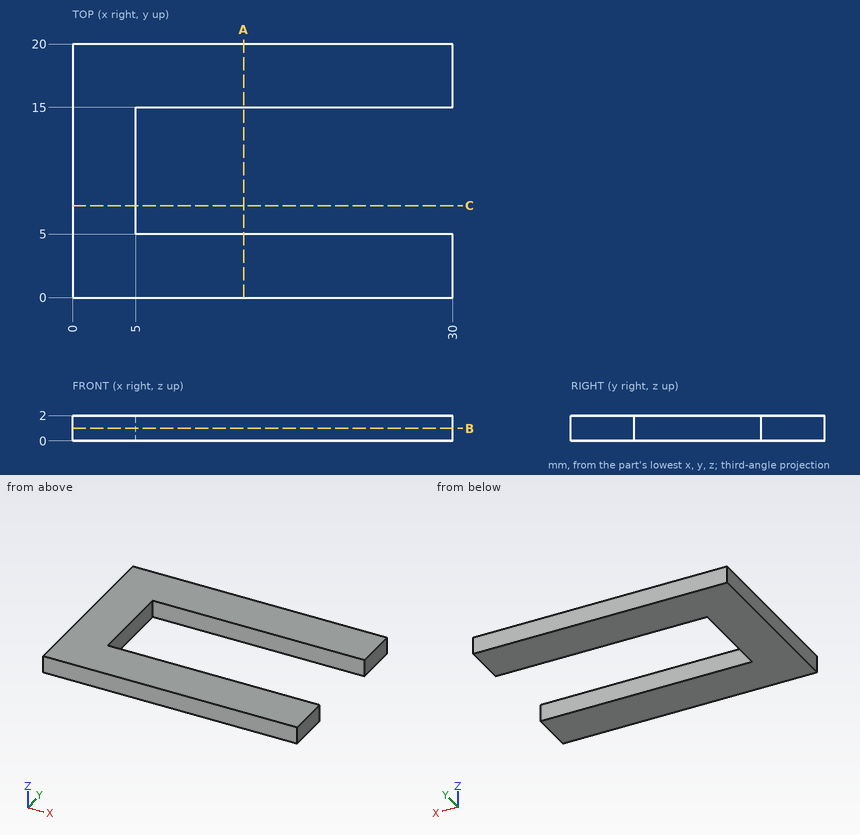
The figure shows three views and two pictorial views of one solid part (mm, origin at its lowest corner). Answer the questions. Coordinates: 2 decimals unless noted, no trailing zeros. Loops run counter-clockwise (first coordinate to the right, second up) from the corner with the lowest first, then second, coordinate; pieces in that order, holes last. Notation, with made-up numbers: M 27,-21.5 L 58,-21.5 A19 cw 58,-3.5 Z; hole C -23.75,51.25 d1. An arc over 180 degrees is marked long. Use CSV: the item, a comma, the result in double quotes. Start each with the question number.
(1) Find section B-B, the plane z = 1. Give the vertices of the cut face in (x, y), then the cut area to 3 significant figures.
(2) Find section A-A, the plane x = 13.5. Give the vertices of the cut face in (y, z), then the cut area to 3 significant figures.
(3) Given pin 1 Ø0.6 at (y, z) = (9.5, 0.5) entering from +X, flat-ended and moving along its own axis, determine where the tip first touches the part or whether it passes through.
(4) Consider line 1 (Y direction, x = 21.75, z = 1.95); line 2 (X direction, y = 11.5, z = 0.65). Determine where each line is inside the solid, lowest interval first.
(5) Find section C-C, the plane y = 7.25. Give the vertices of the cut face in (x, z).
Recorded:
1,outline,"M 0,0 L 30,0 L 30,5 L 5,5 L 5,15 L 30,15 L 30,20 L 0,20 Z"
1,area,"350 mm^2"
2,outline,"M 0,0 L 5,0 L 5,2 L 0,2 Z; M 15,0 L 20,0 L 20,2 L 15,2 Z"
2,area,"20.0 mm^2"
3,pin 1,"stops at x = 5"
4,line 1,"y = 0 to 5, 15 to 20"
4,line 2,"x = 0 to 5"
5,outline,"M 0,0 L 5,0 L 5,2 L 0,2 Z"
